Design review of the part built by this model. Coordinates are the model's own, in mm. Face numbers are marked on the shaded views. Coordinates: 2 decimals unless noted, no trailing zeros. Write each loop counter-clockwise with the first axis right and the second up, starting at its lowest first coordinate (ties: lowest second). Pieces come first, ordered by that corner, then holes. Notation, with made-up numbers: (-14, -4.75) - (27, -4.75) arc R32 cw to (27, 28.25) - close; hole circle Ø7 at (61, -18). An arc over 180 degrees is marked (long way). Use a Markdown table: item, result.
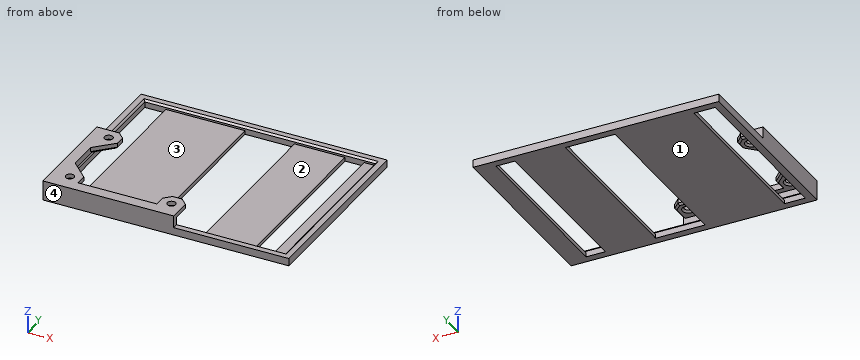
from build123d import *

# Parameters (mm, degrees)
SKETCH002_W     = 64.59
SKETCH002_H     = 49.9
SKETCH002_W_2   = 60.59
SKETCH002_H_2   = 45.9
PAD_DEPTH       = 1
PAD001_DEPTH    = 1.6
SKETCH005_R     = 1.1
PAD002_DEPTH    = 1.6
CHAMFER_SIZE    = 0.49
SKETCH_W        = 64.59
SKETCH_H        = 49.9
SKETCH_W_2      = 13
SKETCH_H_2      = 45.9
SKETCH_W_3      = 5
SKETCH_W_4      = 5.56
PAD003_DEPTH    = 1
CHAMFER001_SIZE = 0.49


with BuildPart() as part:
    # Sketch002 → Pad (new body)
    with BuildSketch(Plane.XY):
        with Locations((32.295, 24.95)):
            Rectangle(SKETCH002_W, SKETCH002_H)
        with Locations((32.295, 24.95)):
            Rectangle(SKETCH002_W_2, SKETCH002_H_2, mode=Mode.SUBTRACT)
    extrude(amount=PAD_DEPTH)

    # Sketch006 (on Face10 of Pad) → Pad001 (join)
    with BuildSketch(Plane.XY.offset(1)):
        Polygon((0, 27.36), (0, 0), (34.34, 0), (34.34, 1.5), (1.5, 1.5), (1.5, 27.36), align=None)
    extrude(amount=PAD001_DEPTH)

    # Sketch005 (on Face17 of Pad001) → Pad002 (join)
    with BuildSketch(Plane.XY.offset(2.6)):
        Polygon((0, 0), (34.34, 0), (34.34, 5.912641), (32.582641, 7.67), (30.097359, 7.67), (28.34, 5.912641), (28.34, 3), (7.67, 3), (7.67, 5.912641), (3, 10.582641), (3, 18.447359), (7.67, 23.117359), (7.67, 25.602641), (5.912641, 27.36), (0, 27.36), align=None)
        with Locations((31.34, 4.67)):
            Circle(SKETCH005_R, mode=Mode.SUBTRACT)
        with Locations((4.67, 24.36)):
            Circle(SKETCH005_R, mode=Mode.SUBTRACT)
        with Locations((4.67, 4.67)):
            Circle(SKETCH005_R, mode=Mode.SUBTRACT)
    extrude(amount=PAD002_DEPTH)

    # Chamfer
    chamfer_edges = [part.edges().sort_by_distance(p)[0] for p in [
        (2, 24.95, 1),
        (32.295, 2, 1),
        (62.59, 24.95, 1),
        (32.295, 47.9, 1),
    ]]
    chamfer(chamfer_edges, length=CHAMFER_SIZE)

    # Sketch (on Face18 of Chamfer) → Pad003 (join)
    with BuildSketch(Plane(origin=(0, 0, 0), x_dir=(1, 0, 0), z_dir=(0, 0, -1))):
        with Locations((32.295, -24.95)):
            Rectangle(SKETCH_W, SKETCH_H)
        with Locations((34.84, -24.95)):
            Rectangle(SKETCH_W_2, SKETCH_H_2, mode=Mode.SUBTRACT)
        with Locations((57.09, -24.95)):
            Rectangle(SKETCH_W_3, SKETCH_H_2, mode=Mode.SUBTRACT)
        with Locations((4.78, -24.95)):
            Rectangle(SKETCH_W_4, SKETCH_H_2, mode=Mode.SUBTRACT)
    extrude(amount=PAD003_DEPTH)

    # Chamfer001
    chamfer001_edges = [part.edges().sort_by_distance(p)[0] for p in [
        (34.34, 3.70632, 2.6),
        (33.46132, 6.79132, 2.6),
        (30.24, 4.67, 2.6),
        (31.34, 7.67, 2.6),
        (29.21868, 6.79132, 2.6),
        (28.34, 4.45632, 2.6),
        (7.67, 4.45632, 2.6),
        (5.335, 8.247641, 2.6),
        (3.70632, 27.36, 2.6),
        (6.79132, 26.48132, 2.6),
        (7.67, 24.36, 2.6),
        (5.335, 20.782359, 2.6),
        (3.57, 4.67, 2.6),
        (3.57, 24.36, 2.6),
    ]]
    chamfer(chamfer001_edges, length=CHAMFER001_SIZE)


solid = part.part
(1) For L1, parallel to X at y = 45, z = -0.25; L2, parallel to Y at x = 34.5, z = -0.5; L3, parallel to Y at x = 4.67, z = 3.4, list the stretches that pass through material, from the lowest coordinate up. Write a range as from..to.
Determined:
| item | result |
|---|---|
| L1 | 0..2, 7.56..28.34, 41.34..54.59, 59.59..64.59 |
| L2 | 0..2, 47.9..49.9 |
| L3 | 0..3.57, 5.77..8.91, 20.12..23.26, 25.46..27.36 |
(2) Take a section at B-B on y = 39.5. Write out the cut boundary in (x, z).
Determined:
| item | result |
|---|---|
| outline | (0, -1) - (2, -1) - (2, 0.51) - (1.51, 1) - (0, 1) - close; (7.56, -1) - (28.34, -1) - (28.34, 0) - (7.56, 0) - close; (41.34, -1) - (54.59, -1) - (54.59, 0) - (41.34, 0) - close; (59.59, -1) - (64.59, -1) - (64.59, 1) - (63.08, 1) - (62.59, 0.51) - (62.59, 0) - (59.59, 0) - close |
(3) For pin 1 (2 mm diameter, centred on x = 54, y = 13, fed in from +Z); pin 2 (0.8 mm diameter, centred on y = 25, z = -0.5, fed in from -X); pin 3 (1.3 mm diameter, centred on y = 12.5, z = 3.5, fed in from +X); pin 4 (1.8 mm diameter, centred on x = 4.67, y = 4.67, fed in from +Z), all flat-tipped, find the tip position at first contact; note any pin that passes through.
Determined:
| item | result |
|---|---|
| pin 1 | z = 0 |
| pin 2 | x = 0 |
| pin 3 | x = 3 |
| pin 4 | through |
(4) Draft analysis for pull direction Y (two halves, no side actions). For the marked faces 1, 2, 3 and 4, state which applies: +Y half, -Y half, draft (parallel to the pull), parting line (faces both ways), or undercut.
Determined:
| item | result |
|---|---|
| face 1 | draft |
| face 2 | undercut |
| face 3 | undercut |
| face 4 | -Y half |
(5) Take a section at C-C on y = 24.36. State how many separate pieces and enclosed holes the cut face has, and give its area (3 significant figures).
Determined:
| item | result |
|---|---|
| separate pieces | 5 |
| enclosed holes | 0 |
| area | 55.6 mm2 |
(6) Take a section at A-A on x = 58.5. Write out the cut boundary in (y, z), and give its area (3 significant figures).
Determined:
| item | result |
|---|---|
| outline | (0, -1) - (2, -1) - (2, 0.51) - (1.51, 1) - (0, 1) - close; (47.9, -1) - (49.9, -1) - (49.9, 1) - (48.39, 1) - (47.9, 0.51) - close |
| area | 7.76 mm2 |
